Check sheet for the modelled part. Datum: model origin and axes. Units: mm. A direction names the side the tool comes from. Coordinates: 2 decimals unless noted, no trailing zeros. Order: outer loops, then holes, each group sorted by start corner. A loop starts at its lowest first (then second) coordinate and runs counter-clockwise, first axis right, second up.
1. Cross-section at A-A (z = 0). Enter the section's corners in (x, y).
2. Cross-section at C-C (y = 26). Enter the section's corners in (x, z), then the cut area to 3 significant figures.
3. Thickness scan on line 1 (X direction, y = 19.5, z = 9.75); line 2 (X direction, y = 1, z = 0); line 3 (Y direction, x = 10, z = -5.5). Record the ranges inside material, lowest first.
4. Cross-section at B-B (y = 19). Enter the section's corners in (x, z).
5. Draft check along Z on faces 1 (the cylindrical face through (-17.729, 23.804, 0.488)), 2 (the flat face through (18, 33, 0)), 3 (the flat face through (0, 2, 10.5)), 4 (the flat face through (0, 2, -10.5)). Enter one of: released by +Z, released by -Z, zero draft, split by the parting line, or undercut.
6. Gauge pin test, flat ends, axial feed: pin 1 Ø2 at (x, z) = (-4, 5.5) entering from -Y; pin 2 Ø5 at (x, z) = (12, 5.5) entering from +Y. Record the tip position at first contact, or that the pin passes through.
7. Cross-section at D-D (x = 11.5). Enter the section's corners in (y, z).
8. Set-up check for faces 5 (the flat face through (-16.25, 18, 0)), 6 (the cylindrical face through (17.771, 23.804, 0.488)): record each of +Z, -Z, +X, -X, +Y, -Y from which the full face is reachable in a straight line by a thin tool's end or side.
```python
from build123d import *

# Parameters (mm, degrees)
SKETCH1_W           = 32.5
SKETCH1_H           = 21
BOSS_EXTRUDE1_DEPTH = 3
SKETCH1_3_W         = 3
SKETCH1_3_H         = 21
BOSS_EXTRUDE2_DEPTH = 33
SKETCH2_R           = 2.25
CUT_EXTRUDE1_DEPTH  = 52.783201909
SKETCH3_R           = 1.5
CUT_EXTRUDE2_DEPTH  = 38.159285515


with BuildPart() as part:
    # Sketch1 → Boss-Extrude1 (new body)
    with BuildSketch(Plane(origin=(0, 0, 0), x_dir=(1, 0, 0), z_dir=(0, 1, 0))):
        Rectangle(SKETCH1_W, SKETCH1_H)
    extrude(amount=BOSS_EXTRUDE1_DEPTH)

    # Sketch1_3 → Boss-Extrude2 (add)
    with BuildSketch(Plane(origin=(0, 0, 0), x_dir=(1, 0, 0), z_dir=(0, 1, 0))):
        with Locations((-17.75, 0)):
            Rectangle(SKETCH1_3_W, SKETCH1_3_H)
        with Locations((17.75, 0)):
            Rectangle(SKETCH1_3_W, SKETCH1_3_H)
    extrude(amount=BOSS_EXTRUDE2_DEPTH)

    # Sketch2 → Cut-Extrude1 (cut, through all)
    with BuildSketch(Plane(origin=(19.25, 0, 0), x_dir=(0, 0, -1), z_dir=(1, 0, 0))):
        with Locations((0, 26)):
            Circle(SKETCH2_R)
    extrude(amount=-CUT_EXTRUDE1_DEPTH, mode=Mode.SUBTRACT)

    # Sketch3 → Cut-Extrude2 (cut, through all)
    with BuildSketch(Plane(origin=(0, 3, 0), x_dir=(1, 0, 0), z_dir=(0, 1, 0))):
        with Locations(Location((0, 0, 0), (0, 0, 270))):
            Circle(SKETCH3_R)
    extrude(amount=-CUT_EXTRUDE2_DEPTH, mode=Mode.SUBTRACT)


solid = part.part
```
Data:
1. outline: (-19.25, 0) - (-1.5, 0) - (-1.5, 3) - (-16.25, 3) - (-16.25, 23.75) - (-19.25, 23.75) - close; (-19.25, 28.25) - (-16.25, 28.25) - (-16.25, 33) - (-19.25, 33) - close; (1.5, 0) - (19.25, 0) - (19.25, 23.75) - (16.25, 23.75) - (16.25, 3) - (1.5, 3) - close; (16.25, 28.25) - (19.25, 28.25) - (19.25, 33) - (16.25, 33) - close
2. outline: (-19.25, -10.5) - (-16.25, -10.5) - (-16.25, -2.25) - (-19.25, -2.25) - close; (-19.25, 2.25) - (-16.25, 2.25) - (-16.25, 10.5) - (-19.25, 10.5) - close; (16.25, -10.5) - (19.25, -10.5) - (19.25, -2.25) - (16.25, -2.25) - close; (16.25, 2.25) - (19.25, 2.25) - (19.25, 10.5) - (16.25, 10.5) - close
2. area: 99.0 mm2
3. line 1: x = -19.25 to -16.25, 16.25 to 19.25
3. line 2: x = -19.25 to -1.5, 1.5 to 19.25
3. line 3: y = 0 to 3
4. outline: (-19.25, -10.5) - (-16.25, -10.5) - (-16.25, 10.5) - (-19.25, 10.5) - close; (16.25, -10.5) - (19.25, -10.5) - (19.25, 10.5) - (16.25, 10.5) - close
5. face 1: undercut
5. face 2: zero draft
5. face 3: released by +Z
5. face 4: released by -Z
6. pin 1: stops at y = 0
6. pin 2: stops at y = 3
7. outline: (0, -10.5) - (3, -10.5) - (3, 10.5) - (0, 10.5) - close
8. face 5: +Z, -Z, +Y
8. face 6: +X, -X
